For this review, take the finished solid that the model builds, in its own axes (mm). A direction names the side the tool comes from. Coordinates: 2 decimals unless noted, no trailing zeros. Write each loop counter-clockwise with the first axis right and the second up, starting at its lowest first coordinate (ties: lowest second). Pieces come first, ordered by that corner, then holes. Notation, with made-up numbers: M 88.25,44.5 L 92.25,44.5 A18 cw 92.25,73.5 Z; hole C 32.25,82.25 d3. An arc over 180 degrees is marked long. One line per question, with ' | ' between items.
from build123d import *

# Parameters (mm, degrees)
ESBO_O1_R                = 22.5
RESSALTO_EXTRUS_O1_DEPTH = 4
CHANFRO1_SIZE            = 2
CORTE_EXTRUS_O1_DEPTH    = 33.070235422
ESBO_O3_R                = 4
CORTE_EXTRUS_O2_DEPTH    = 33.070235422
ESBO_O4_R                = 4.5
CORTE_EXTRUS_O3_DEPTH    = 2
PADR_OCIRCULAR1_COUNT    = 15
ESBO_O5_R                = 20.5
ESBO_O5_R_2              = 18.5
CORTE_EXTRUS_O4_DEPTH    = 1
FURO_ROSCADO_DE_M1_61_D  = 1.25
PADR_OCIRCULAR2_COUNT    = 3


with BuildPart() as part:
    # Esboço1 → Ressalto-extrusão1 (new body)
    with BuildSketch(Plane.XY):
        Circle(ESBO_O1_R)
    extrude(amount=RESSALTO_EXTRUS_O1_DEPTH)

    # Chanfro1
    chanfro1_edges = [part.edges().sort_by_distance(p)[0] for p in [
        (-22.5, 0, 4),
    ]]
    chamfer(chanfro1_edges, length=CHANFRO1_SIZE)

    # Esboço2 → Corte-extrusão1 (cut, through all)
    with BuildSketch(Plane(origin=(0, 0, 0), x_dir=(-1, 0, 0), z_dir=(0, 0, -1))):
        with BuildLine():
            Line((1.75, -22.431841208), (1.75, -14.931841208))
            ThreePointArc((1.75, -14.931841208), (0, -13.181841208), (-1.75, -14.931841208))
            Line((-1.75, -14.931841208), (-1.75, -22.431841208))
            ThreePointArc((-1.75, -22.431841208), (0, -22.5), (1.75, -22.431841208))
        make_face()
    corte_extrus_o1 = extrude(amount=-CORTE_EXTRUS_O1_DEPTH, mode=Mode.SUBTRACT)

    # Esboço3 → Corte-extrusão2 (cut, through all)
    with BuildSketch(Plane(origin=(0, 0, 0), x_dir=(-1, 0, 0), z_dir=(0, 0, -1))):
        Circle(ESBO_O3_R)
    extrude(amount=-CORTE_EXTRUS_O2_DEPTH, mode=Mode.SUBTRACT)

    # Esboço4 → Corte-extrusão3 (cut)
    with BuildSketch(Plane(origin=(0, 0, 0), x_dir=(-1, 0, 0), z_dir=(0, 0, -1))):
        Circle(ESBO_O4_R)
    extrude(amount=-CORTE_EXTRUS_O3_DEPTH, mode=Mode.SUBTRACT)

    # PadrãoCircular1: Corte-extrusão1 ×15 about axis
    padr_ocircular1_axis = Axis((0, 0, 0), (0, 0, 1))
    for i in range(1, PADR_OCIRCULAR1_COUNT):
        add(corte_extrus_o1.rotate(padr_ocircular1_axis, i * 360 / PADR_OCIRCULAR1_COUNT), mode=Mode.SUBTRACT)

    # Esboço5 → Corte-extrusão4 (cut)
    with BuildSketch(Plane(origin=(0, 0, 0), x_dir=(-1, 0, 0), z_dir=(0, 0, -1))):
        Circle(ESBO_O5_R)
        Circle(ESBO_O5_R_2, mode=Mode.SUBTRACT)
    extrude(amount=-CORTE_EXTRUS_O4_DEPTH, mode=Mode.SUBTRACT)

    # Furo roscado de M1.61 (through all)
    with Locations(Plane(origin=(0, 6, 0), x_dir=(-1, 0, 0), z_dir=(0, 0, -1))):
        with Locations((0, 0)):
            furo_roscado_de_m1_61 = Hole(FURO_ROSCADO_DE_M1_61_D / 2)

    # PadrãoCircular2: Furo roscado de M1.61 ×3 about axis
    padr_ocircular2_axis = Axis((0, 0, 0), (0, 0, 1))
    for i in range(1, PADR_OCIRCULAR2_COUNT):
        add(furo_roscado_de_m1_61.rotate(padr_ocircular2_axis, i * 360 / PADR_OCIRCULAR2_COUNT), mode=Mode.SUBTRACT)


solid = part.part
1) The part is to be moulded in two halves that separate along Y. For faces 4 (the cylindrical face through (-9.822, -8.792, 1.972)), 5 (the conical face through (-12.661, -17.359, 3.014)), 6 (the cylindrical face through (0, 22.5, 1)), say which applies: +Y half, -Y half, draft (parallel to the pull), parting line (faces both ways), or undercut.
Responses:
face 4: undercut | face 5: -Y half | face 6: +Y half
2) We need section B-B on z = 2.75. State how many separate pieces and enclosed holes the cut face has, then the cut area to 3 significant figures.
Responses:
separate pieces: 1 | enclosed holes: 4 | area: 1,000 mm^2
3) To check wall thickness, follow line 1 along Y through (x, z) = (16, 0.7); line 2 along Y through (x, z) = (-13.5, 0.4); line 3 along Y through (x, z) = (20, 1.85). State the ranges of each line that lie inside material, in increasing order. Write a range as [from, to].
Responses:
line 1: [-9.29, -7.04], [-3.36, -0.08], [3.44, 7.22], [12.82, 15.82] | line 2: [-18, -15.43], [-9.8, -6.22], [-3.01, 0.45], [2.67, 5.81], [9.81, 12.65], [15.43, 15.6] | line 3: [-10.31, -8.34], [-4.66, 0.34], [3.86, 9.53]
4) Insertion check: pin 1 Ø0.7 at (x, y) = (-19.5, -3) entering from -Z; pin 2 Ø2 at (x, z) = (-5, 0.5) entering from -Y; pin 3 Ø1 at (x, z) = (-4, 3) entering from -Y. Each pin has a flat end and moves straight along its axis. Give the tip position at first contact, or say it passes through.
Responses:
pin 1: z = 1 | pin 2: y = -22.14 | pin 3: y = -21.64
5) Machinability: for faces 1 (the flat face through (17, -10, 1)), 2 (the cylindrical face through (9.77, -8.85, 1.97)), 3 (the flat face through (-18.45, 3.7, 1.97)), which of the approach directions +Z, -Z, +X, -X, +Y, -Y give a long, thin tool a straight path to every point of the face, cutting with its end or side? Answer none if there is none.
Responses:
face 1: -Z | face 2: +Z, -Z | face 3: +Z, -Z, -X
6) We need section A-A on x = 0. State the section outline as (y, z) points (3 decimals), then the cut area to 3 significant figures.
Responses:
outline: M -13.182,0 L -4.5,0 L -4.5,2 L -4,2 L -4,4 L -13.182,4 Z; M 4,2 L 4.5,2 L 4.5,0 L 5.375,0 L 5.375,4 L 4,4 Z; M 6.625,0 L 18.5,0 L 18.5,1 L 20.5,1 L 20.5,0 L 22.5,0 L 22.5,2 L 20.5,4 L 6.625,4 Z | area: 99.7 mm^2
